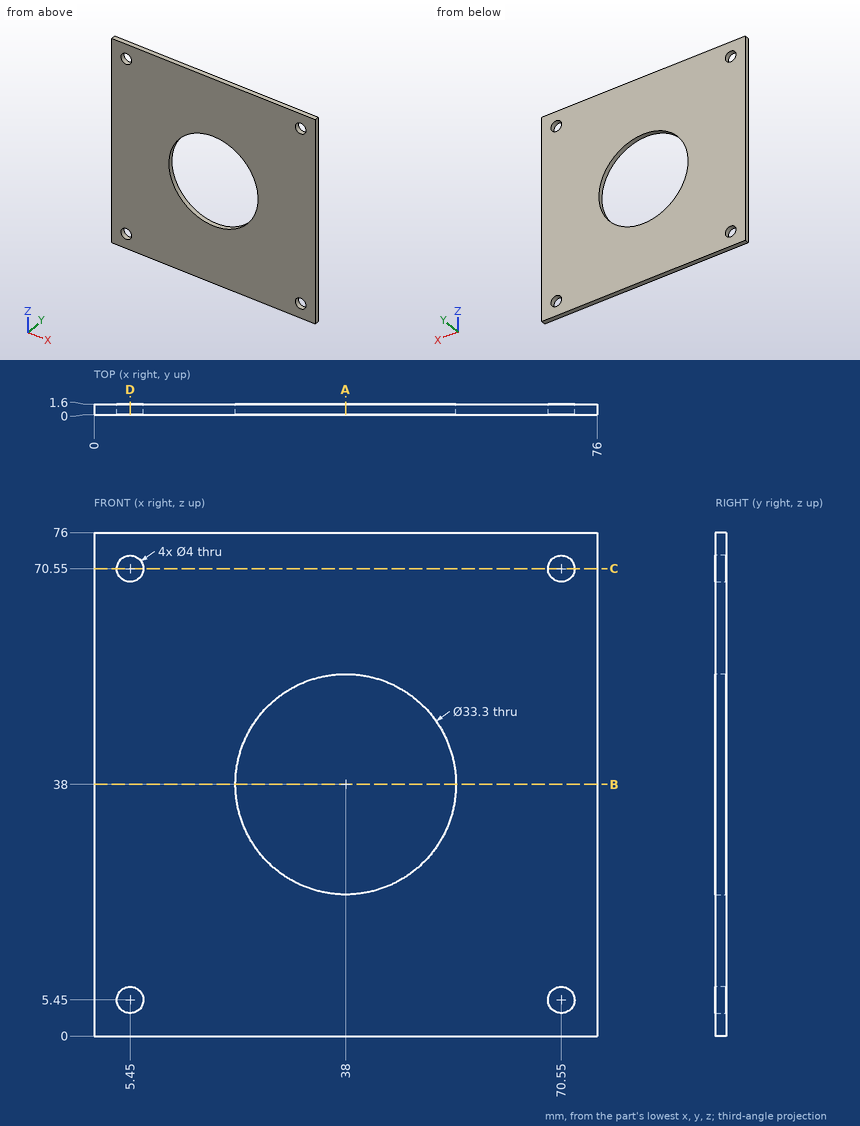
Could you check a few things on this drawing? It's one solid part, dimensions in mm from its lowest x, y, z. Give positions to 0.01 mm unless a question says otherwise; leave off trailing zeros. Order: outer loops, then holes, each group sorted by start corner. A loop starts at its lowest first (then second) coordinate and runs counter-clockwise, first axis right, second up. Notation, with made-up numbers: (38.5, -10) - (96.5, -10) arc R34 ccw to (96.5, 29) - close; hole circle Ø1 at (55, 12). An arc over 180 degrees is marked (long way). Answer as a JSON object with one key per item and string values. Group by question number.
Item 1: If we section it at B-B on z = 38: Please give me the cut outline in (x, y).
Item 2: For P1, Ø2.5, axis at x = 5.45, z = 5.45, coming from the -Y side; P2, Ø4.5, axis at x = 70.55, z = 5.45, coming from the +Y side, each with a flat end and sliding along its axis, tell me the tip position at first contact or that it passes through.
Item 3: Please list where these lines run through material, in increasing order: probe 1 along X at (y, z) = (1.2, 70.55); probe 2 along X at (y, z) = (1.15, 38); probe 3 along Z at (x, y) = (4.5, 0.15).
Item 4: If we section it at A-A on x = 38: Please give me the cut outline in (y, z), and give its area (3 significant figures).
Item 5: If we section it at D-D on x = 5.45: Please give me the cut outline in (y, z), and give its area (3 significant figures).
Item 6: If we section it at C-C on z = 70.55: Please give me the cut outline in (x, y), and give its area (3 significant figures).
Result set:
{
 "1": {"outline": "(0, 0) - (21.35, 0) - (21.35, 1.6) - (0, 1.6) - close; (54.65, 0) - (76, 0) - (76, 1.6) - (54.65, 1.6) - close"},
 "2": {"P1": "through", "P2": "y = 1.6"},
 "3": {"probe 1": "0 to 3.45, 7.45 to 68.55, 72.55 to 76", "probe 2": "0 to 21.35, 54.65 to 76", "probe 3": "0 to 3.69, 7.21 to 68.79, 72.31 to 76"},
 "4": {"outline": "(0, 0) - (1.6, 0) - (1.6, 21.35) - (0, 21.35) - close; (0, 54.65) - (1.6, 54.65) - (1.6, 76) - (0, 76) - close", "area": "68.3 mm²"},
 "5": {"outline": "(0, 0) - (1.6, 0) - (1.6, 3.45) - (0, 3.45) - close; (0, 7.45) - (1.6, 7.45) - (1.6, 68.55) - (0, 68.55) - close; (0, 72.55) - (1.6, 72.55) - (1.6, 76) - (0, 76) - close", "area": "109 mm²"},
 "6": {"outline": "(0, 0) - (3.45, 0) - (3.45, 1.6) - (0, 1.6) - close; (7.45, 0) - (68.55, 0) - (68.55, 1.6) - (7.45, 1.6) - close; (72.55, 0) - (76, 0) - (76, 1.6) - (72.55, 1.6) - close", "area": "109 mm²"}
}
